Work out the finished part from the listing and answer in its coordinate system (mm). A direction names the side the tool comes from. Coordinates: 2 decimals unless noted, no trailing zeros. Loops run counter-clockwise (first coordinate to the right, second up) from the corner with the lowest first, then second, coordinate; pieces in that order, holes last. Notation, with made-up numbers: (42, 21) - (82, 21) arc R32 ccw to (82, 60) - close; hole circle Ø2 at (41.25, 16.25). An arc over 180 degrees is marked (long way). Write each question's results on one line, items separated by ' | '. Start each with the question number.
Item 1: Section B-B, the plane z = 0 is taken. Write down the section's boundary in (x, y).
Item 2: Section C-C, the plane y = 50 is taken. Write down the section's boundary in (x, z), plus the area to 3 significant figures.
Item 3: Consider probe 1 along Y at (x, z) = (-0.6, -1.7); probe 2 along Z at (x, y) = (-0.35, 69); probe 3 along X at (y, z) = (63, 0.9). Determine where each line is inside the solid, lowest interval first. Write a range as [from, to].
Item 4: For a pull along Y with two mould halves and no side action, classify faces 5 (the face through (1.3, 11, -1.3)), 6 (the face through (0, 0, 0)), 7 (the face through (0, 102, 0)) as +Y half, -Y half, draft (parallel to the pull), parting line (faces both ways), or undercut.
Item 5: A tool of negligible diameter and unlimited length cuts with its end or side. For faces 1 (the face through (-0.07, 62.48, 1.5)), 2 (the face through (0, 36, 3)), 3 (the face through (-0.07, 100.48, 1.5)), 4 (the face through (-0.07, 1.48, 1.5)), from which of +Z, -Z, +X, -X, +Y, -Y can it reach the whole face along a straight path? Write none if from no direction.
Item 6: Section A-A, the plane x = 0 is taken. Write down the section's boundary in (y, z).
from build123d import *


with BuildPart() as part:
    # Sketch1 → Revolve1 (revolve)
    with BuildSketch(Plane(origin=(0, 0, 0), x_dir=(0, 0, -1), z_dir=(1, 0, 0))):
        Polygon((0, 102), (1.5, 102), (1.5, 99), (3, 99), (3, 64), (1.5, 64), (1.5, 61), (3, 61), (3, 11), (1.5, 11), (1.5, 8), (3, 8), (3, 3), (1.5, 3), (1.5, 0), (0, 0), align=None)
    revolve(axis=Axis((0, 0, 0), (0, 1, 0)))


solid = part.part
Answer key:
1) outline: (-3, 3) - (-1.5, 3) - (-1.5, 0) - (1.5, 0) - (1.5, 3) - (3, 3) - (3, 8) - (1.5, 8) - (1.5, 11) - (3, 11) - (3, 61) - (1.5, 61) - (1.5, 64) - (3, 64) - (3, 99) - (1.5, 99) - (1.5, 102) - (-1.5, 102) - (-1.5, 99) - (-3, 99) - (-3, 64) - (-1.5, 64) - (-1.5, 61) - (-3, 61) - (-3, 11) - (-1.5, 11) - (-1.5, 8) - (-3, 8) - close
2) outline: circle Ø6 at (0, 0) | area: 28.3 mm^2
3) probe 1: y = [3, 8], [11, 61], [64, 99] | probe 2: z = [-2.98, 2.98] | probe 3: x = [-1.2, 1.2]
4) face 5: undercut | face 6: -Y half | face 7: +Y half
5) face 1: none | face 2: +Y, -Y | face 3: +Y | face 4: -Y
6) outline: (0, -1.5) - (3, -1.5) - (3, -3) - (8, -3) - (8, -1.5) - (11, -1.5) - (11, -3) - (61, -3) - (61, -1.5) - (64, -1.5) - (64, -3) - (99, -3) - (99, -1.5) - (102, -1.5) - (102, 1.5) - (99, 1.5) - (99, 3) - (64, 3) - (64, 1.5) - (61, 1.5) - (61, 3) - (11, 3) - (11, 1.5) - (8, 1.5) - (8, 3) - (3, 3) - (3, 1.5) - (0, 1.5) - close
